Check sheet for the modelled part. Datum: model origin and axes. Units: mm. Face numbers are marked on the shaded views. A direction names the side the tool comes from. Round coordinates to 2 decimals unless told otherwise and drop trailing zeros. Write each loop counter-clockwise with the first axis right and the second up, starting at its lowest first coordinate (ties: lowest second). Pieces come first, ordered by that corner, then holes.
Item 1: Material ranges on line 1 (X direction, y = 843, z = 0); line 2 (X direction, y = 752, z = 0); line 3 (Z direction, x = -4, y = 884), recorded low to high.
Item 2: Cross-section at C-C on y = 539.5. Enter the section's corners in (x, z), plus the area to 3 significant figures.
Item 3: Cross-section at A-A on x = 0. Enter the section's corners in (y, z), plus the area to 3 significant figures.
Item 4: Cross-section at B-B on z = 0. Enter the section's corners in (x, y).
Item 5: Go/stop test with flat-tipped pins: pin 1 Ø6 at (x, y) = (22, 300) entering from +Z; pin 2 Ø12 at (x, y) = (-27, 568.5) entering from -Z; pin 3 Ø2 at (x, y) = (-41, 233) entering from -Z. Record where each tip stops, or that it passes through.
Item 6: Tool access check on the marked faces 1 and 2. Record the directions out of +Z, -Z, +X, -X, +Y, -Y that give a thin tool (end or side, any length) a straight path to the whole face; none if there is none.
Item 7: Release check for a two-part mould opening along Z. For the marked faces 3 and 4 record: +Z half, -Z half, draft (parallel to the pull), parting line (faces both ways), or undercut.
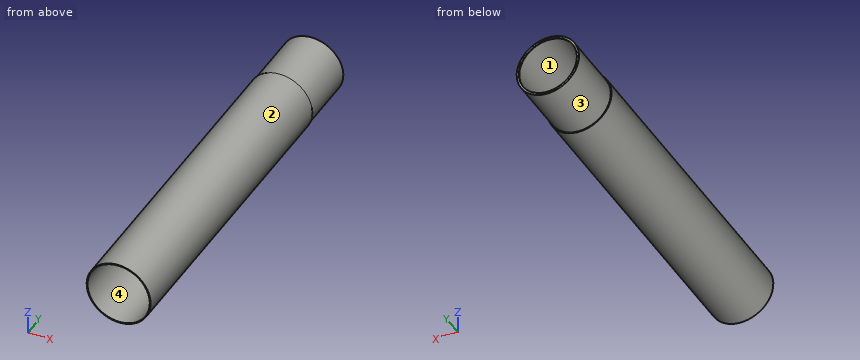
from build123d import *

# Parameters (mm, degrees)
SKETCH1_W                = 1.96
SKETCH1_H                = 774
BOSS_EXTRUDE1_DEPTH      = 152
BOSS_EXTRUDE1_DEPTH_BACK = 152
SKETCH3_R                = 76.2
SKETCH3_R_2              = 75.2
BOSS_EXTRUDE2_START      = -2
SKETCH4_R                = 76.2
SKETCH4_R_2              = 70.915017824
BOSS_EXTRUDE2_DEPTH      = 2


with BuildPart() as part:
    # Sketch1 → Revolve1 (revolve)
    with BuildSketch(Plane.XY, mode=Mode.PRIVATE) as revolve1_sk:
        with Locations((77.18, 387)):
            Rectangle(SKETCH1_W, SKETCH1_H)
    revolve(revolve1_sk.sketch.rotate(Axis((0, 204.615384615, 0), (0, -1, 0)), 90), axis=Axis((0, 204.615384615, 0), (0, -1, 0)))

    # Sketch3 → Boss-Extrude1 (add, two sides: drawn at the far end of the back side and taken through both)
    with BuildSketch(Plane(origin=(0, 774, 0), x_dir=(1, 0, 0), z_dir=(0, 1, 0)).offset(-BOSS_EXTRUDE1_DEPTH_BACK)):
        with Locations(Location((0, 0, 0), (0, 0, 270))):
            Circle(SKETCH3_R)
        with Locations(Location((0, 0, 0), (0, 0, 270))):
            Circle(SKETCH3_R_2, mode=Mode.SUBTRACT)
    extrude(amount=BOSS_EXTRUDE1_DEPTH + BOSS_EXTRUDE1_DEPTH_BACK)

    # Sketch4 → Boss-Extrude2 (add)
    with BuildSketch(Plane(origin=(0, 926, 0), x_dir=(1, 0, 0), z_dir=(0, 1, 0)).offset(BOSS_EXTRUDE2_START)):
        with Locations(Location((0, 0, 0), (0, 0, 270))):
            Circle(SKETCH4_R)
        with Locations(Location((0, 0, 0), (0, 0, 270))):
            Circle(SKETCH4_R_2, mode=Mode.SUBTRACT)
    extrude(amount=BOSS_EXTRUDE2_DEPTH)


solid = part.part
Response values:
1. line 1: x = -76.2 to -75.2, 75.2 to 76.2
1. line 2: x = -78.16 to -75.2, 75.2 to 78.16
1. line 3: z = -76.09 to -75.09, 75.09 to 76.09
2. outline: circle Ø156.32 at (0, 0); hole circle Ø152.4 at (0, 0)
2. area: 950 mm2
3. outline: (0, -78.16) - (774, -78.16) - (774, -76.2) - (926, -76.2) - (926, -70.92) - (924, -70.92) - (924, -75.2) - (622, -75.2) - (622, -76.2) - (0, -76.2) - close; (0, 76.2) - (622, 76.2) - (622, 75.2) - (924, 75.2) - (924, 70.92) - (926, 70.92) - (926, 76.2) - (774, 76.2) - (774, 78.16) - (0, 78.16) - close
3. area: 3,660 mm2
4. outline: (-78.16, 0) - (-76.2, 0) - (-76.2, 622) - (-75.2, 622) - (-75.2, 924) - (-70.92, 924) - (-70.92, 926) - (-76.2, 926) - (-76.2, 774) - (-78.16, 774) - close; (70.92, 924) - (75.2, 924) - (75.2, 622) - (76.2, 622) - (76.2, 0) - (78.16, 0) - (78.16, 774) - (76.2, 774) - (76.2, 926) - (70.92, 926) - close
5. pin 1: stops at z = 75.82
5. pin 2: stops at z = -75.29
5. pin 3: stops at z = -67.15
6. face 1: -Y
6. face 2: +Y, -Y
7. face 3: parting line
7. face 4: undercut
